```python
from build123d import *

# Parameters (mm, degrees)
SKETCH_W    = 95
SKETCH_H    = 62
PAD_DEPTH   = 890
FILLET_R    = 20
FILLET001_R = 12


with BuildPart() as part:
    # Sketch → Pad (new body)
    with BuildSketch(Plane.YZ):
        with Locations((47.5, 31)):
            Rectangle(SKETCH_W, SKETCH_H)
    extrude(amount=PAD_DEPTH)

    # Fillet
    fillet_edges = [part.edges().sort_by_distance(p)[0] for p in [
        (0, 0, 31),
        (890, 0, 31),
        (890, 95, 31),
        (0, 95, 31),
    ]]
    fillet(fillet_edges, radius=FILLET_R)

    # Fillet001
    fillet001_edges = [part.edges().sort_by_distance(p)[0] for p in [
        (445, 95, 62),
        (5.857864, 89.142136, 62),
        (884.142136, 89.142136, 62),
        (0, 47.5, 62),
        (890, 47.5, 62),
        (5.857864, 5.857864, 62),
        (884.142136, 5.857864, 62),
        (445, 0, 62),
    ]]
    fillet(fillet001_edges, radius=FILLET001_R)


solid = part.part
```
Geometry: final body of the model. Coordinates: model frame, mm. Coordinates: 2 decimals unless noted, no trailing zeros. Use CSV: the item, a comma, the result in double quotes.
1) Line query: line 1 (Y direction, x = 699.5, z = 51); line 2 (X direction, y = 45, z = 56); line 3 (X direction, y = 6, z = 44). Output: solid intervals per line, ascending.
Findings:
line 1,"y = 0.04 to 94.96"
line 2,"x = 1.61 to 888.39"
line 3,"x = 5.72 to 884.28"
2) Pin query (flat end, axial travel): pin 1 Ø5 at (y, z) = (83.5, 38) entering from +X. Return the tip coordinate at first contact, or that it passes through.
Findings:
pin 1,"stops at x = 889.08"
3) Mould query, pull axis Z, two halves, no side actions, for faces 1 (the flat face through (439, 47, 0)), 2 (the cylindrical face through (883.986, 89.297, 25.35)), 3 (the flat face through (439, 47, 62)). Classes: +Z half, -Z half, draft (parallel to the pull), parting line (faces both ways), or undercut.
Findings:
face 1,"-Z half"
face 2,"draft"
face 3,"+Z half"
